For this review, take the finished solid that the model builds, in its own axes (mm). A direction names the side the tool comes from. Round coordinates to 2 decimals unless told otherwise and drop trailing zeros. Order: outer loops, then holes, each group sorted by start corner. A loop starts at its lowest first (then second) coordinate and runs counter-clockwise, first axis right, second up.
from build123d import *

# Parameters (mm, degrees)
BOSS_EXTRU_1_DEPTH    = 10
BOSS_EXTRU_1_2_DEPTH  = 10
BOSS_EXTRU_1_3_DEPTH  = 10
BOSS_EXTRU_1_4_DEPTH  = 10
BOSS_EXTRU_1_5_DEPTH  = 10
BOSS_EXTRU_1_6_DEPTH  = 10
BOSS_EXTRU_1_7_DEPTH  = 10
BOSS_EXTRU_1_8_DEPTH  = 10
BOSS_EXTRU_1_9_DEPTH  = 10
BOSS_EXTRU_1_10_DEPTH = 10
BOSS_EXTRU_1_11_DEPTH = 10
BOSS_EXTRU_1_12_DEPTH = 10
BOSS_EXTRU_1_13_DEPTH = 10
ESQUISSE2_W           = 22
ESQUISSE2_H           = 17
BOSS_EXTRU_2_DEPTH    = 9


with BuildPart() as part:
    # Esquisse1 → Boss.-Extru.1 (new body)
    with BuildSketch(Plane.XY):
        Polygon((5.443717547, 11.812499229), (3.550061207, 6.914484272), (4.023475292, 6.914484272), (5.443717547, 10.587995489), (6.172046909, 8.462184165), (6.554419824, 8.899181782), align=None)
    extrude(amount=BOSS_EXTRU_1_DEPTH)



with BuildPart() as body_2:
    # Esquisse1 → Boss.-Extru.1 2 (new body)
    with BuildSketch(Plane.XY):
        with BuildLine():
            Line((6.902626833, 8.065470566), (5.678236467, 6.71845465))
            ThreePointArc((5.678236467, 6.71845465), (6.407694377, 6.234618767), (6.902626833, 5.512643789))
            Line((6.902626833, 5.512643789), (8.09044996, 4.808141168))
            Line((8.09044996, 4.808141168), (6.902626833, 8.065470566))
        make_face()
    extrude(amount=BOSS_EXTRU_1_2_DEPTH)


with BuildPart() as body_3:
    # Esquisse1 → Boss.-Extru.1 3 (new body)
    with BuildSketch(Plane.XY):
        Polygon((7.496538396, 9.023251364), (4.987277184, 6.289858676), (5.776031703, 7.600137795), (7.245503612, 9.363504086), (6.902626833, 9.649234735), (8.09044996, 9.988029647), (7.698590784, 8.65325933), align=None)
    extrude(amount=BOSS_EXTRU_1_3_DEPTH)


with BuildPart() as body_4:
    # Esquisse1 → Boss.-Extru.1 4 (new body)
    with BuildSketch(Plane.XY):
        with BuildLine():
            ThreePointArc((19.283756817, 7.855107538), (19.571781089, 7.751485217), (19.70217296, 7.474549255))
            Line((19.70217296, 7.474549255), (19.70217296, 5.694123098))
            Line((19.70217296, 5.694123098), (19.357163158, 5.694123098))
            Line((19.357163158, 5.694123098), (19.357163158, 7.183832057))
            ThreePointArc((19.357163158, 7.183832057), (19.328585973, 7.343227565), (19.195669208, 7.435730089))
            Line((19.195669208, 7.435730089), (18.601077847, 7.435730089))
            Line((18.601077847, 7.435730089), (18.601077847, 5.694123098))
            Line((18.601077847, 5.694123098), (18.270749313, 5.694123098))
            Line((18.270749313, 5.694123098), (18.270749313, 7.855107538))
            Line((18.270749313, 7.855107538), (19.283756817, 7.855107538))
        make_face()
    extrude(amount=BOSS_EXTRU_1_4_DEPTH)


with BuildPart() as body_5:
    # Esquisse1 → Boss.-Extru.1 5 (new body)
    with BuildSketch(Plane.XY):
        with BuildLine():
            Line((16.494479646, 7.435730089), (16.494479646, 6.027121876))
            ThreePointArc((16.494479646, 6.027121876), (16.601754173, 5.813714283), (16.828510675, 5.738666872))
            Line((16.828510675, 5.738666872), (17.640470987, 5.738666872))
            ThreePointArc((17.640470987, 5.738666872), (17.880768825, 5.838201495), (17.980303448, 6.078499332))
            Line((17.980303448, 6.078499332), (17.980303448, 7.435730089))
            ThreePointArc((17.980303448, 7.435730089), (17.896289803, 7.716195302), (17.638564331, 7.855107538))
            Line((17.638564331, 7.855107538), (16.828516054, 7.855107538))
            ThreePointArc((16.828516054, 7.855107538), (16.574641936, 7.714600019), (16.494479646, 7.435730089))
        make_face()
        with BuildLine():
            Line((17.638564331, 7.273362699), (17.638564331, 6.215464578))
            ThreePointArc((17.638564331, 6.215464578), (17.633763509, 6.142841489), (17.599745165, 6.078499332))
            Line((17.599745165, 6.078499332), (16.929772089, 6.078499332))
            ThreePointArc((16.929772089, 6.078499332), (16.85077764, 6.126011144), (16.828516054, 6.215464578))
            Line((16.828516054, 6.215464578), (16.828516054, 7.273362699))
            ThreePointArc((16.828516054, 7.273362699), (16.85715067, 7.368261985), (16.929772089, 7.435730089))
            Line((16.929772089, 7.435730089), (17.537308296, 7.435730089))
            ThreePointArc((17.537308296, 7.435730089), (17.621563701, 7.375517206), (17.638564331, 7.273362699))
        make_face(mode=Mode.SUBTRACT)
    extrude(amount=BOSS_EXTRU_1_5_DEPTH)


with BuildPart() as body_6:
    # Esquisse1 → Boss.-Extru.1 6 (new body)
    with BuildSketch(Plane.XY):
        with BuildLine():
            ThreePointArc((15.811686316, 7.435730089), (15.697522048, 7.386612234), (15.651527288, 7.271154337))
            Line((15.651527288, 7.271154337), (15.651527288, 5.738666872))
            Line((15.651527288, 5.738666872), (15.345769144, 5.738666872))
            Line((15.345769144, 5.738666872), (15.345769144, 7.435730089))
            ThreePointArc((15.345769144, 7.435730089), (15.440912126, 7.720805224), (15.709766935, 7.855107538))
            Line((15.709766935, 7.855107538), (16.328563178, 7.855107538))
            Line((16.328563178, 7.855107538), (16.328563178, 7.435730089))
            Line((16.328563178, 7.435730089), (15.811686316, 7.435730089))
        make_face()
    extrude(amount=BOSS_EXTRU_1_6_DEPTH)


with BuildPart() as body_7:
    # Esquisse1 → Boss.-Extru.1 7 (new body)
    with BuildSketch(Plane.XY):
        with BuildLine():
            Line((14.161212762, 8.462184165), (14.161212762, 6.076587297))
            ThreePointArc((14.161212762, 6.076587297), (14.270058526, 5.833555854), (14.518873285, 5.738672251))
            Line((14.518873285, 5.738672251), (15.09368484, 5.738672251))
            Line((15.09368484, 5.738672251), (15.09368484, 6.076587297))
            Line((15.09368484, 6.076587297), (14.659382776, 6.076587297))
            ThreePointArc((14.659382776, 6.076587297), (14.560703645, 6.116109364), (14.518873285, 6.213832369))
            Line((14.518873285, 6.213832369), (14.518873285, 7.435730089))
            Line((14.518873285, 7.435730089), (15.09368484, 7.435730089))
            Line((15.09368484, 7.435730089), (15.09368484, 7.855107538))
            Line((15.09368484, 7.855107538), (14.518873285, 7.855107538))
            Line((14.518873285, 7.855107538), (14.518873285, 8.462184165))
            Line((14.518873285, 8.462184165), (14.161212762, 8.462184165))
        make_face()
    extrude(amount=BOSS_EXTRU_1_7_DEPTH)


with BuildPart() as body_8:
    # Esquisse1 → Boss.-Extru.1 8 (new body)
    with BuildSketch(Plane.XY):
        with BuildLine():
            ThreePointArc((13.886262231, 6.102623129), (13.805699319, 5.85605539), (13.574383017, 5.738672251))
            Line((13.574383017, 5.738672251), (12.738992267, 5.738672251))
            Line((12.738992267, 5.738672251), (12.738992267, 4.808141168))
            Line((12.738992267, 4.808141168), (12.338004706, 4.808141168))
            Line((12.338004706, 4.808141168), (12.338004706, 7.295933822))
            ThreePointArc((12.338004706, 7.295933822), (12.422689818, 7.658567923), (12.738992267, 7.855107538))
            Line((12.738992267, 7.855107538), (13.574383017, 7.855107538))
            ThreePointArc((13.574383017, 7.855107538), (13.817178537, 7.710011113), (13.886262231, 7.435730089))
            Line((13.886262231, 7.435730089), (13.886262231, 6.102623129))
        make_face()
        with BuildLine():
            Line((13.574383017, 7.295933822), (13.574383017, 6.213832369))
            ThreePointArc((13.574383017, 6.213832369), (13.502737587, 6.119010995), (13.38502778, 6.102623129))
            Line((13.38502778, 6.102623129), (12.738992267, 6.102623129))
            Line((12.738992267, 6.102623129), (12.738992267, 7.295933822))
            ThreePointArc((12.738992267, 7.295933822), (12.749024413, 7.381980031), (12.81696207, 7.435730089))
            Line((12.81696207, 7.435730089), (13.38502778, 7.435730089))
            ThreePointArc((13.38502778, 7.435730089), (13.508658154, 7.405048709), (13.574383017, 7.295933822))
        make_face(mode=Mode.SUBTRACT)
    extrude(amount=BOSS_EXTRU_1_8_DEPTH)


with BuildPart() as body_9:
    # Esquisse1 → Boss.-Extru.1 9 (new body)
    with BuildSketch(Plane.XY):
        with BuildLine():
            Line((10.727068381, 7.446462813), (11.468195577, 7.446462813))
            ThreePointArc((11.468195577, 7.446462813), (11.596758234, 7.435730089), (11.705162978, 7.365787542))
            Line((11.705162978, 7.365787542), (11.705162978, 7.043119919))
            Line((11.705162978, 7.043119919), (10.888410557, 7.043119919))
            ThreePointArc((10.888410557, 7.043119919), (10.530519911, 6.390896085), (10.888410557, 5.738672251))
            Line((10.888410557, 5.738672251), (12.047997327, 5.738672251))
            Line((12.047997327, 5.738672251), (12.047997327, 7.514651407))
            ThreePointArc((12.047997327, 7.514651407), (11.948280035, 7.755390246), (11.707541196, 7.855107538))
            Line((11.707541196, 7.855107538), (10.727068381, 7.855107538))
            Line((10.727068381, 7.855107538), (10.727068381, 7.446462813))
        make_face()
        with BuildLine():
            ThreePointArc((11.097631979, 6.65067692), (10.91259355, 6.376650024), (11.097631979, 6.102623129))
            Line((11.097631979, 6.102623129), (11.705154613, 6.102623129))
            Line((11.705154613, 6.102623129), (11.705154613, 6.65067692))
            Line((11.705154613, 6.65067692), (11.097631979, 6.65067692))
        make_face(mode=Mode.SUBTRACT)
    extrude(amount=BOSS_EXTRU_1_9_DEPTH)


with BuildPart() as body_10:
    # Esquisse1 → Boss.-Extru.1 10 (new body)
    with BuildSketch(Plane.XY):
        with BuildLine():
            Line((8.533065369, 5.73880671), (9.772658698, 5.73880671))
            ThreePointArc((9.772658698, 5.73880671), (10.174227228, 5.895270347), (10.34754256, 6.289858676))
            Line((10.34754256, 6.289858676), (10.34754256, 7.944071011))
            ThreePointArc((10.34754256, 7.944071011), (10.206978339, 8.417727517), (9.772658698, 8.65325933))
            Line((9.772658698, 8.65325933), (8.533065369, 8.65325933))
            Line((8.533065369, 8.65325933), (8.533065369, 5.73880671))
        make_face()
        with BuildLine():
            ThreePointArc((9.772658698, 6.102623129), (9.919227173, 6.151592523), (9.988240146, 6.289858676))
            Line((9.988240146, 6.289858676), (9.988240146, 7.944071011))
            ThreePointArc((9.988240146, 7.944071011), (9.912548031, 8.115618007), (9.772658698, 8.240472493))
            Line((9.772658698, 8.240472493), (8.892367783, 8.240472493))
            Line((8.892367783, 8.240472493), (8.892367783, 6.102623129))
            Line((8.892367783, 6.102623129), (9.772658698, 6.102623129))
        make_face(mode=Mode.SUBTRACT)
    extrude(amount=BOSS_EXTRU_1_10_DEPTH)


with BuildPart() as body_11:
    # Esquisse1 → Boss.-Extru.1 11 (new body)
    with BuildSketch(Plane.XY):
        Polygon((4.355542191, 5.73880671), (4.464623497, 6.213832369), (3.265683859, 6.289858676), (2.677895095, 4.808141168), (3.633556258, 5.286480868), align=None)
    extrude(amount=BOSS_EXTRU_1_11_DEPTH)


with BuildPart() as body_12:
    # Esquisse1 → Boss.-Extru.1 12 (new body)
    with BuildSketch(Plane.XY):
        Polygon((4.199345564, 6.972570668), (5.173183133, 9.229859022), (4.987277184, 7.680642785), (5.678236467, 7.944071011), (4.560132448, 5.83905846), (4.868736322, 7.227775894), align=None)
    extrude(amount=BOSS_EXTRU_1_12_DEPTH)


with BuildPart() as body_13:
    # Esquisse1 → Boss.-Extru.1 13 (new body)
    with BuildSketch(Plane.XY):
        with BuildLine():
            Line((4.49284458, 6.389276558), (3.344161613, 6.46328358))
            Line((3.344161613, 6.46328358), (3.204994268, 6.426280069))
            ThreePointArc((3.204994268, 6.426280069), (2.812494667, 6.690009625), (3.265683859, 6.825023594))
            Line((3.265683859, 6.825023594), (3.396366031, 6.71845465))
            Line((3.396366031, 6.71845465), (4.291345624, 6.71845465))
            Line((4.291345624, 6.71845465), (4.640038971, 6.914484272))
            Line((4.640038971, 6.914484272), (4.49284458, 6.389276558))
        make_face()
    extrude(amount=BOSS_EXTRU_1_13_DEPTH)


with BuildPart() as part_1:
    add(part.part)

    add(body_2.part)  # Boss.-Extru.2 merges body 2

    add(body_3.part)  # Boss.-Extru.2 merges body 3

    add(body_4.part)  # Boss.-Extru.2 merges body 4

    add(body_5.part)  # Boss.-Extru.2 merges body 5

    add(body_6.part)  # Boss.-Extru.2 merges body 6

    add(body_7.part)  # Boss.-Extru.2 merges body 7

    add(body_8.part)  # Boss.-Extru.2 merges body 8

    add(body_9.part)  # Boss.-Extru.2 merges body 9

    add(body_10.part)  # Boss.-Extru.2 merges body 10

    add(body_11.part)  # Boss.-Extru.2 merges body 11

    add(body_12.part)  # Boss.-Extru.2 merges body 12

    add(body_13.part)  # Boss.-Extru.2 merges body 13
    # Esquisse2 → Boss.-Extru.2 (add)
    with BuildSketch(Plane.XY):
        with Locations((11, 8.5)):
            Rectangle(ESQUISSE2_W, ESQUISSE2_H)
    extrude(amount=BOSS_EXTRU_2_DEPTH)


solid = part_1.part
(1) Tool access review of faces 4 (the face through (6.9, 8.6, 10)), 5 (the face through (4.724, 8.726, 9.493)), 6 (the face through (6.4, 6.24, 9.49)): name each direction out of +Z, -Z, +X, -X, +Y, -Y from which nothing blocks a thin tool from reaching the whole face with its end or side.
(2) Wall thickness on L1, parallel to Z at x = 9, y = 8: over which ranges is the line inside the solid? List them lowest first.
(3) Add section A-A on x = 1.5. Give the boundary of the cut face in (y, z), plus the area to 3 significant figures.
(4) Clearance check with flat-ended pins moving along their axes: P1, Ø0.8, axis at y = 6.5, z = 9.5, coming from the -X side; P2, Ø0.5, axis at x = 15, z = 9.5, coming from the +Y side; P3, Ø0.6, axis at x = 15, z = 9.5, coming from the -Y side. State where each tip first meets the part, or that it passes through.
(5) Add section B-B on y = 13.5. Give the boundary of the cut face in (x, z), plus the area to 3 significant figures.
(6) Draft analysis for pull direction X (two halves, no side actions). For faces 1 (the face through (13.2, 5.739, 9.5)), 2 (the face through (17.2, 7.855, 9.5)), 3 (the face through (4.51, 9.4, 9.49)), state which applies: pulls with the +X half, pulls with the -X half, needs draft (parallel to the pull), parting line crosses it, or undercut.
Here are the results:
1. face 4: +Z, +X, -X, +Y, -Y
1. face 5: +Z
1. face 6: +Z, -Y
2. L1: z = 0 to 9
3. outline: (0, 0) - (17, 0) - (17, 9) - (0, 9) - close
3. area: 153 mm2
4. P1: stops at x = 2.81
4. P2: stops at y = 7.86
4. P3: stops at y = 5.74
5. outline: (0, 0) - (22, 0) - (22, 9) - (0, 9) - close
5. area: 198 mm2
6. face 1: undercut
6. face 2: needs draft
6. face 3: pulls with the -X half
